Can you work these out from the drawing? Everything is in mm from the part's minimum corner. A direction names the side the tool comes from. Round coordinates to 2 decimals unless told otherwise and drop trailing zeros. Loops run counter-clockwise (first coordinate to the right, second up) from the corner with the lowest first, then second, coordinate; pieces in that order, holes last. Notation, with made-up numbers: (42.5, 14) - (58.5, 14) arc R14 ccw to (58.5, 25) - close; hole circle Ø10 at (61, 54.25). An arc over 180 degrees is marked (long way). Put each result on its own line as item: value. Start each with the question number.
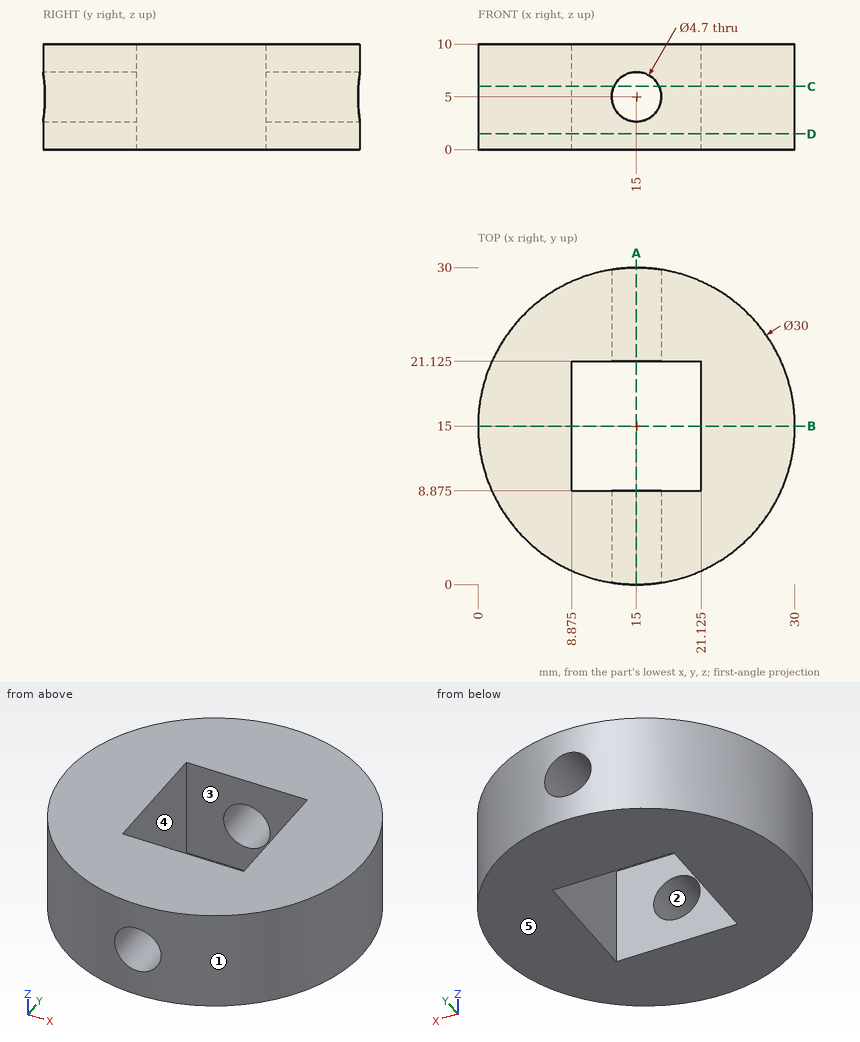
Item 1: Suppose I cut it at C-C, the plane z = 6. List the corners of the cut face in (x, y) for me (3 decimals).
Item 2: Suppose I cut it at B-B, the plane y = 15. List the corners of the cut face in (x, z) for me (3 decimals), then the cut area to 4 significant figures.
Item 3: Will these pins go through, and if not, where does the flat tip stop? P1, Ø3, axis at y = 4, z = 6, coming from the -X side; P2, Ø2, axis at x = 12.5, z = 7, coming from the -Y side; P3, Ø3, axis at y = 4.5, z = 4.5, coming from the +X side.
Item 4: On a 3-axis mill with a long thin cutter (end or side, diameter ignored), from which of +Z, -Z, +X, -X, +Y, -Y can I reach the whole of each face in a straight line? I mean the marked faces 4 and 5. Say none if no direction works.
Item 5: Suppose I cut it at D-D, the plane z = 1.5. List the corners of the cut face in (x, y) for me (3 decimals).
Item 6: Thinking about a two-plate mould opening in Y: for the marked faces 1, 2 and 3, which applies, released by +Y, released by -Y, zero draft, split by the parting line, or undercut?
Item 7: Suppose I cut it at A-A, the plane x = 15. List the corners of the cut face in (y, z) for me (3 decimals).
Item 8: I need wall thicknesses on line 1 (X direction, y = 14, z = 7.75) (3 decimals); line 2 (X direction, y = 5.5, z = 5.5); line 3 (Z direction, x = 17, y = 5.5). Which ranges of each line are inside material? Lowest first, please. Write a range as from..to.
Numbers:
1. outline: (8.875, 8.875) - (8.875, 21.125) - (12.873, 21.125) - (12.873, 29.848) arc R15 ccw to (12.873, 0.152) - (12.873, 8.875) - close; (17.127, 0.152) arc R15 ccw to (17.127, 29.848) - (17.127, 21.125) - (21.125, 21.125) - (21.125, 8.875) - (17.127, 8.875) - close
2. outline: (0, 0) - (8.875, 0) - (8.875, 10) - (0, 10) - close; (21.125, 0) - (30, 0) - (30, 10) - (21.125, 10) - close
2. area: 177.5 mm^2
3. P1: x = 3.39
3. P2: y = 0.08
3. P3: x = 27
4. face 4: +Z, -Z
4. face 5: -Z, +X, -X, +Y, -Y
5. outline: circle Ø30 at (15, 15); hole (8.875, 8.875) - (21.125, 8.875) - (21.125, 21.125) - (8.875, 21.125) - close
6. face 1: split by the parting line
6. face 2: zero draft
6. face 3: undercut
7. outline: (0, 0) - (8.875, 0) - (8.875, 2.65) - (0, 2.65) - close; (0, 7.35) - (8.875, 7.35) - (8.875, 10) - (0, 10) - close; (21.125, 0) - (30, 0) - (30, 2.65) - (21.125, 2.65) - close; (21.125, 7.35) - (30, 7.35) - (30, 10) - (21.125, 10) - close
8. line 1: 0.033..8.875, 21.125..29.967
8. line 2: 3.39..12.7, 17.3..26.61
8. line 3: 0..3.77, 6.23..10
